The drawing under review shows one solid part. Ordinate dimensions are in mm from its lowest x, y, z. Coordinates: 2 decimals unless noted, no trailing zeros. Loops run counter-clockwise (first coordinate to the right, second up) from the corner with the lowest first, then second, coordinate; pieces in that order, holes last. Notation, with made-up numbers: (-2.75, -7) - (2.25, -7) arc R29 cw to (2.25, 28) - close; hole circle Ø7 at (21.25, 28.5). An arc over 180 degrees is marked (long way). Use one line per item in the form item = value. Start each with the question number.
1. For pin 1 Ø10 at (x, y) = (8.5, 7) entering from +Z (1 decimal); pin 2 Ø5.5 at (y, z) = (20, 53) entering from -X; pin 3 Ø1.2 at (x, y) = (12.7, 6.35) entering from -Z; pin 4 Ø4.5 at (y, z) = (4.78, 53.98) entering from -X (1 decimal), all flat-tipped, find the tip position at first contact; note any pin that passes through.
2. Add section B-B on y = 15.5. Give the boundary of the cut face in (x, z) (1 decimal), and give its area (3 significant figures).
3. Add section D-D on y = 24. Give the boundary of the cut face in (x, z) (1 decimal).
4. Draft analysis for pull direction Z (two halves, no side actions). For the marked faces 1, 2, 3 and 4, state which applies: +Z half, -Z half, draft (parallel to the pull), parting line (faces both ways), or undercut.
5. Add section A-A on x = 3. Give the boundary of the cut face in (y, z).
6. To check wall thickness, follow probe 1 along Z at (x, y) = (22, 4.75) (1 decimal); probe 2 along Z at (x, y) = (16, 13) (1 decimal); probe 3 along Z at (x, y) = (20.25, 5.75) (1 decimal). State the ranges of each line that lie inside material, in increasing order.
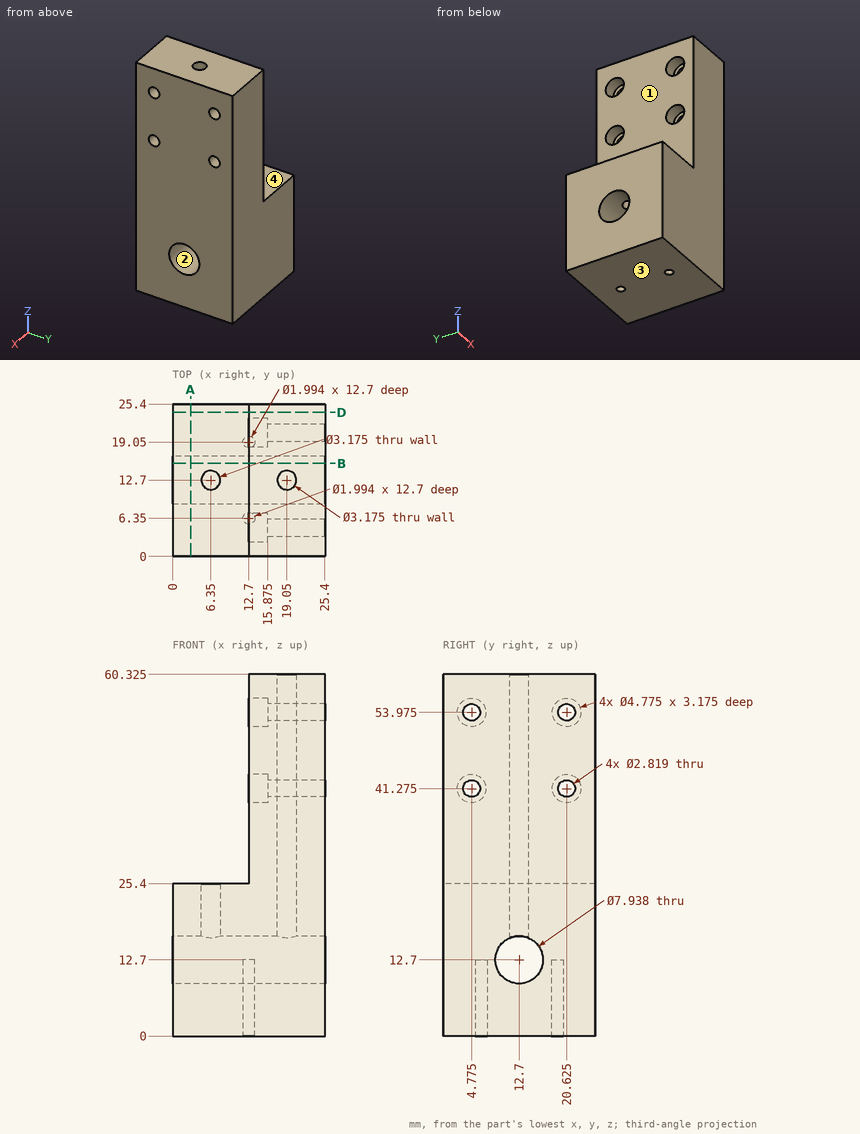
Conclusion:
q1.pin_1 = 60.3
q1.pin_2 = 12.7
q1.pin_3 = 12.7
q1.pin_4 = 15.9
q2.outline = (0, 0) - (25.4, 0) - (25.4, 9.9) - (0, 9.9) - close; (0, 15.5) - (25.4, 15.5) - (25.4, 60.3) - (12.7, 60.3) - (12.7, 25.4) - (0, 25.4) - close
q2.area = 946 mm^2
q3.outline = (0, 0) - (25.4, 0) - (25.4, 60.3) - (12.7, 60.3) - (12.7, 25.4) - (0, 25.4) - close
q4.face_1 = draft
q4.face_2 = undercut
q4.face_3 = -Z half
q4.face_4 = +Z half
q5.outline = (0, 0) - (25.4, 0) - (25.4, 25.4) - (0, 25.4) - close; hole circle Ø7.94 at (12.7, 12.7)
q6.probe_1 = 0 to 39.9, 42.7 to 52.6, 55.4 to 60.3
q6.probe_2 = 0 to 8.7, 16.7 to 60.3
q6.probe_3 = 0 to 40.3, 42.3 to 53, 55 to 60.3
